Model file for the job. Use its own axes, mm. A direction names the side the tool comes from. Coordinates: 2 decimals unless noted, no trailing zeros. Order: outer loops, then holes, each group sorted by start corner. A loop starts at its lowest first (then second) coordinate and runs counter-clockwise, first axis right, second up.
from build123d import *

# Parameters (mm, degrees)
MAIN_DEPTH          = 9.75
SKETCH4_R           = 6.5
BASECIRCLE_DEPTH    = 1
SKETCH5_R           = 3
GEAR_DEPTH          = 4.8
SKETCH9_R           = 2.25
FIXING_HOLE_DEPTH   = 19.05
FIXINGFILLET_R      = 2
REINFORCEMENT_DEPTH = 0.5
SERVOFILLET_R       = 0.5


with BuildPart() as part:
    # Sketch1 → Main (new body, symmetric)
    with BuildSketch(Plane(origin=(0, 0, 0), x_dir=(0, 0, -1), z_dir=(1, 0, 0))):
        Polygon((-40.5, 0), (0, 0), (0, 29), (6.65, 29), (6.65, 32.5), (0, 32.5), (0, 36.3), (-5.8, 36.3), (-5.8, 39), (-40.5, 39), (-40.5, 32.5), (-47.15, 32.5), (-47.15, 29), (-40.5, 29), align=None)
    extrude(amount=MAIN_DEPTH, both=True)

    # Sketch4 → BaseCircle (add)
    with BuildSketch(Plane(origin=(0, 39, 0), x_dir=(1, 0, 0), z_dir=(0, 1, 0))):
        with Locations((0, -31.2)):
            Circle(SKETCH4_R)
    extrude(amount=BASECIRCLE_DEPTH)

    # Sketch5 → Gear (add)
    with BuildSketch(Plane(origin=(0, 40, 0), x_dir=(1, 0, 0), z_dir=(0, 1, 0))):
        with Locations((0, -31.2)):
            Circle(SKETCH5_R)
    extrude(amount=GEAR_DEPTH)

    # Sketch9 → Fixing-Hole (cut)
    with BuildSketch(Plane(origin=(0, 32.5, 0), x_dir=(-1, 0, 0), z_dir=(0, 1, 0))):
        with Locations((-4.75, 45)):
            Circle(SKETCH9_R)
        with Locations((4.75, 45)):
            Circle(SKETCH9_R)
        with Locations((4.75, -4.5)):
            Circle(SKETCH9_R)
        with Locations((-4.75, -4.5)):
            Circle(SKETCH9_R)
    extrude(amount=-FIXING_HOLE_DEPTH, mode=Mode.SUBTRACT)

    # FixingFillet
    fixingfillet_edges = [part.edges().sort_by_distance(p)[0] for p in [
        (-9.75, 30.75, 47.15),
        (9.75, 30.75, -6.65),
        (-9.75, 30.75, -6.65),
        (9.75, 30.75, 47.15),
    ]]
    fillet(fixingfillet_edges, radius=FIXINGFILLET_R)

    # Esquisse1 → Reinforcement (add, symmetric)
    with BuildSketch(Plane(origin=(0, 0, 0), x_dir=(0, 0, -1), z_dir=(1, 0, 0))):
        Polygon((6.65, 32.5), (0, 34), (0, 32.5), align=None)
        Polygon((-47.15, 32.5), (-40.5, 32.5), (-40.5, 34), align=None)
    extrude(amount=REINFORCEMENT_DEPTH, both=True)

    # ServoFillet
    servofillet_edges = [part.edges().sort_by_distance(p)[0] for p in [
        (9.75, 14.5, 0),
        (-9.75, 14.5, 0),
        (-9.75, 14.5, 40.5),
        (9.75, 14.5, 40.5),
    ]]
    fillet(servofillet_edges, radius=SERVOFILLET_R)


solid = part.part
Q1. Drop flat-ended pins along their axis: P1, Ø3.5, axis at x = -3.5, z = 44, coming from the +Y side; P2, Ø1.5, axis at x = 3, y = 12, coming from the +Z side; P3, Ø1, axis at x = -1.5, z = 15.5, coming from the +Y side. Give the stop position or say it passes through.
Established:
P1: stops at y = 32.5
P2: stops at z = 40.5
P3: stops at y = 39
Q2. Cut at C-C, the plane x = 4.75. List the corners of the cut face in (y, z).
Established:
outline: (0, 0) - (29, 0) - (29, -2.25) - (32.5, -2.25) - (32.5, 0) - (36.3, 0) - (36.3, 5.8) - (39, 5.8) - (39, 26.76) - (40, 26.76) - (40, 35.64) - (39, 35.64) - (39, 40.5) - (32.5, 40.5) - (32.5, 42.75) - (29, 42.75) - (29, 40.5) - (0, 40.5) - close
Q3. Which spindle directions (+Z, -Z, +X, -X, +Y, -Y) get a long thin tool onto all of the face, cutting with end or side? Do faces 4 (the face through (3, 40, 33)), 5 (the face through (0.1, 34.4, 0)), 6 (the face through (6.2, 32.5, 43)), 7 (the face through (0, 15, 40.5)), 8 (the face through (0, 36.3, 3)). Say none if no direction does.
Established:
face 4: +Y
face 5: -Z, +Y
face 6: +Z, +X, +Y
face 7: +Z, +X, -X, -Y
face 8: -Z, +X, -X, +Y
Q4. Cut at D-D, the plane y = 30.5. List the corners of the cut face in (x, z), plus the area to 3 significant figures.
Established:
outline: (-9.75, -4.65) arc R2 ccw to (-7.75, -6.65) - (-5.41, -6.65) arc R2.25 cw (long way) to (-4.09, -6.65) - (4.09, -6.65) arc R2.25 cw (long way) to (5.41, -6.65) - (7.75, -6.65) arc R2 ccw to (9.75, -4.65) - (9.75, 45.15) arc R2 ccw to (7.75, 47.15) - (5.41, 47.15) arc R2.25 cw (long way) to (4.09, 47.15) - (-4.09, 47.15) arc R2.25 cw (long way) to (-5.41, 47.15) - (-7.75, 47.15) arc R2 ccw to (-9.75, 45.15) - close
area: 982 mm2
Q5. Cut at A-A, the plane y = 7.5. List the corners of the cut face in (x, z), plus the area to 3 significant figures.
Established:
outline: (-9.75, 0.5) arc R0.5 ccw to (-9.25, 0) - (9.25, 0) arc R0.5 ccw to (9.75, 0.5) - (9.75, 40) arc R0.5 ccw to (9.25, 40.5) - (-9.25, 40.5) arc R0.5 ccw to (-9.75, 40) - close
area: 790 mm2
Q6. Probe line 1 (X direction, y = 30.55, z = -4.5); line 2 (Y direction, x = -8, z = 24); line 3 (Z direction, x = -5.5, y = 22). List the from-to ranges inside material, lowest first.
Established:
line 1: x = -9.75 to -7, -2.5 to 2.5, 7 to 9.75
line 2: y = 0 to 39
line 3: z = 0 to 40.5
Q7. Mould opens along X. For faces 1 (the face through (4.84, 30.77, 42.75)), 2 (the face through (-9.75, 20, 21)), 3 (the face through (0, 29, 44)) say: pulls with the +X half, pulls with the -X half, needs draft (parallel to the pull), parting line crosses it, or undercut.
Established:
face 1: undercut
face 2: pulls with the -X half
face 3: needs draft
Q8. Cut at B-B, the plane z = 31.2. List the corners of the cut face in (x, y).
Established:
outline: (-9.75, 0) - (9.75, 0) - (9.75, 39) - (6.5, 39) - (6.5, 40) - (3, 40) - (3, 44.8) - (-3, 44.8) - (-3, 40) - (-6.5, 40) - (-6.5, 39) - (-9.75, 39) - close
